Here's how the part is built. I have some questions about the finished solid (model axes, mm). A direction names the side the tool comes from. Coordinates: 2 decimals unless noted, no trailing zeros. Write each loop counter-clockwise with the first axis right and the second up, starting at its lowest first coordinate (ties: lowest second). Pieces come first, ordered by that corner, then holes.
(1) For pin 1 Ø2.5 at (y, z) = (14, 27.51) entering from -X; pin 2 Ø10 at (x, y) = (10.5, 16.5) entering from +Z; pin 3 Ø8 at (x, z) = (12, -0.5) entering from +Y; pin 4 Ø8 at (x, y) = (-25, 17.5) entering from +Z, each with a flat end and sliding along its axis, tell me the tip position at first contact or that it passes through.
(2) Imagine slicing it at D-D, the plane x = 17. List the corners of the cut face in (y, z) for me.
(3) Thinking about a two-plate mould opening in X: for faces 4 (the flat face through (29, 9, 46)), 5 (the flat face through (32.5, 18, 15)), 6 (the flat face through (-16, 4, 17.5)), which applies, released by +X, released by -X, zero draft, split by the parting line, or undercut?
(4) Imagine slicing it at B-B, the plane z = 21. List the corners of the cut face in (x, y) for me.
(5) Please list where these lines run through material, in increasing order: probe 1 along Y at (x, z) = (29.5, 34.5); probe 2 along Y at (x, z) = (-9.5, -12); probe 3 along X at (y, z) = (4.5, 18.5).
(6) Which directions (+Z, -Z, +X, -X, +Y, -Y) give clear straight access to the entire face, cutting with the end or side of a thin tool? Please do faces 1 (the flat face through (-29, 10, 37.5)), 2 (the flat face through (0, 7, -20)), 3 (the flat face through (29, 35, 6.5)).
(7) Imagine slicing it at A-A, the plane y = 19.5. List the corners of the cut face in (x, z) for me, plus the area to 3 significant figures.
(8) Imagine slicing it at C-C, the plane y = 42. List the corners of the cut face in (x, z) for me.
Autodesk Inventor part; units mm, degrees
ref_plane "YZ Plane" through (0, 0, 0) normal (1, 0, 0) x (0, 1, 0)
ref_plane "XZ Plane" through (0, 0, 0) normal (0, 1, 0) x (-1, 0, 0)
ref_plane "XY Plane" through (0, 0, 0) normal (0, 0, 1) x (1, 0, 0)
sketch "Sketch1" plane through (0, 0, 0) normal (0, 1, 0) x (-1, 0, 0)
  line L0 (32.5, 37.5) -> (-32.5, 37.5)
  line L1 (-32.5, 37.5) -> (-32.5, -37.5)
  line L2 (-32.5, -37.5) -> (32.5, -37.5)
  line L3 (32.5, -37.5) -> (32.5, 37.5)
  line L4 (32.5, 37.5) -> (-32.5, -37.5) construction
  line L5 (-32.5, 37.5) -> (32.5, -37.5) construction
  point P0 (0, 0)
  dimension "d0" = 65
  dimension "d1" = 75
extrude "Extrusion1" add sketch "Sketch1" along normal blind 7
sketch "Sketch6" plane through (0, 7, 0) normal (0, 1, 0) x (1, 0, 0)
  line L0 (-32.5, 37.5) -> (-32.5, -37.5)
  line L1 (-32.5, -37.5) -> (-25.5, -37.5)
  line L2 (-32.5, -37.5) -> (32.5, -37.5)
  line L3 (-25.5, -37.5) -> (-25.5, -17.5)
  line L4 (-25.5, -17.5) -> (-5.5, -17.5)
  line L5 (-5.5, -17.5) -> (-5.5, -37.5)
  line L6 (-25.5, -17.5) -> (-32.5, -17.5)
  point P0 (0, 0)
  dimension "d13" = 7
  dimension "d14" = 20
  dimension "d15" = 20
  dimension "d16" = 20
  dimension "d17" = 90
extrude "Extrusion4" cut sketch "Sketch6" against normal blind 14 contours L4 L5 L2 L3
sketch "Sketch7" plane through (0, 7, 0) normal (0, 1, 0) x (1, 0, 0)
  line L0 (-25.5, -37.5) -> (-25.5, -17.5)
  line L1 (-32.5, -37.5) -> (-25.5, -37.5)
  line L2 (-25.5, -37.5) -> (-25.5, -17.5)
  line L3 (-25.5, -17.5) -> (-32.5, -17.5)
  line L4 (-32.5, -17.5) -> (-32.5, -37.5)
  point P0 (0, 0)
extrude "Extrusion5" add sketch "Sketch7" along normal blind 14
sketch "Sketch8" plane through (0, 7, 0) normal (0, 1, 0) x (1, 0, 0)
  line L0 (-5.5, -37.5) -> (32.5, -37.5)
  line L1 (32.5, -37.5) -> (25.5, -37.5)
  line L2 (25.5, -37.5) -> (25.5, 0.5)
  line L3 (25.5, 0.5) -> (32.5, 0.5)
  line L4 (32.5, 0.5) -> (32.5, -37.5)
  point P0 (0, 0)
  dimension "d22" = 7
  dimension "d23" = 38
extrude "Extrusion6" add sketch "Sketch8" along normal blind 18
sketch "Sketch9" plane through (0, 25, 0) normal (0, 1, 0) x (1, 0, 0)
  line L0 (32.5, 0.5) -> (25.5, 0.5)
  line L1 (25.5, 0.5) -> (25.5, -37.5)
  line L2 (32.5, 0.5) -> (25.5, 0.5)
  line L3 (25.5, 0.5) -> (25.5, -6.5)
  line L4 (25.5, -6.5) -> (32.5, -6.5)
  line L5 (32.5, -6.5) -> (32.5, 0.5)
  point P0 (0, 0)
  dimension "d26" = 7
extrude "Extrusion7" add sketch "Sketch9" along normal blind 20
sketch "Sketch10" plane through (0, 25, 0) normal (0, 1, 0) x (1, 0, 0)
  line L0 (32.5, -6.5) -> (32.5, 0.5)
  line L1 (32.5, 0.5) -> (32.5, -54.5)
  line L2 (32.5, -54.5) -> (25.5, -54.5)
  line L3 (25.5, -54.5) -> (25.5, -47.5)
  line L4 (25.5, -47.5) -> (32.5, -47.5)
  line L5 (32.5, -47.5) -> (32.5, -54.5)
  point P0 (0, 0)
  dimension "d29" = 55
  dimension "d30" = 7
  dimension "d31" = 7
extrude "Extrusion8" add sketch "Sketch10" along normal blind 20
sketch "Sketch11" plane through (32.5, 0, 37.5) normal (1, 0, 0) x (0, 0, -1)
  line L0 (-17, 25) -> (-10, 25)
  line L1 (0, 7) -> (0, 25) construction
  line L2 (0, 7) -> (0, 25)
  line L3 (0, 25) -> (-17, 25)
  line L4 (-17, 25) -> (-17, 45)
  line L5 (0, 7) -> (0, 0)
  line L6 (-17, 25) -> (-17, 18)
  line L7 (-17, 18) -> (0, 0)
  point P0 (37.5, 0)
  dimension "d37" = 7
extrude "Extrusion9" add sketch "Sketch11" against normal up to surface (7 mm away)
sketch "Sketch13" plane through (32.5, 0, -37.5) normal (0, 0, -1) x (-1, 0, 0)
  line L0 (65, 7) -> (58, 7)
  line L1 (0, 0) -> (65, 0)
  line L2 (65, 0) -> (65, 7)
  line L3 (65, 7) -> (0, 7)
  line L4 (0, 7) -> (0, 0)
  point P0 (32.5, 0)
extrude "Extrusion10" add sketch "Sketch13" along normal blind 20
sketch "Sketch14" plane through (0, 7, 0) normal (0, 1, 0) x (1, 0, 0)
  point P0 (0, 0)
sketch "Sketch15" plane through (-25.5, 0, 37.5) normal (1, 0, 0) x (0, 0, -1)
  point P0 (37.5, 0)
sketch "Sketch16" plane through (-32.5, 0, 37.5) normal (-1, 0, 0) x (0, 0, 1)
  point P0 (-37.5, 0)
ref_plane "Work Plane1" through (-15.5, 0, 37.5) normal (1, 0, 0) x (0, 0, -1)
mirror "Mirror1" about plane through (-15.5, 0, 37.5) normal (1, 0, 0) of "Extrusion5"
sketch "Sketch18" plane through (-32.5, 0, 37.5) normal (-1, 0, 0) x (0, 0, 1)
  line L0 (-20, 7) -> (-20, 0)
  line L1 (-20, 7) -> (-20, 14)
  line L2 (-20, 7) -> (-20, 21)
  line L3 (-20, 7) -> (-13, 7) construction
  line L4 (-20, 14) -> (-27, 7)
  line L5 (-20, 7) -> (-95, 7)
  point P0 (-37.5, 0)
  dimension "d43" = 7
  dimension "d44" = 90
  dimension "d45" = 45
extrude "Extrusion12" add sketch "Sketch18" against normal up to surface (7 mm away)
mirror "Mirror2" about plane through (-15.5, 0, 37.5) normal (1, 0, 0) of "Extrusion12"
sketch "Sketch19" plane through (-32.5, 0, 37.5) normal (-1, 0, 0) x (0, 0, 1)
  line L0 (0, 0) -> (0, 21)
  line L1 (-20, 14) -> (-20, 21)
  circle A0 centre (-10, 14) radius 1.7 construction
  circle A1 centre (-10, 7) radius 1.7 construction
  point P0 (-37.5, 0)
  dimension "d52" = 3.4
  dimension "d53" = 3.4
sketch "Sketch20" plane through (-32.5, 0, 37.5) normal (-1, 0, 0) x (0, 0, 1)
  line L0 (0, 7) -> (-38, 7)
  circle A0 centre (-9.9905, 7) radius 1.7
  circle A1 centre (-9.9905, 13.9998) radius 1.7
  point P0 (-37.5, 0)
  dimension "d54" = 3.4
  dimension "d55" = 3.4
extrude "Extrusion13" cut sketch "Sketch20" against normal up to surface (34 mm away)
properties part number "graber thingie"
Recorded:
1. pin 1: stops at x = 25.5
1. pin 2: passes through
1. pin 3: stops at y = 7
1. pin 4: stops at z = 37.5
2. outline: (0, -57.5) - (7, -57.5) - (7, 37.5) - (0, 37.5) - close
3. face 4: zero draft
3. face 5: released by +X
3. face 6: undercut
4. outline: (-32.5, 0) - (-25.5, 0) - (-25.5, 21) - (-32.5, 21) - close; (-5.5, 0) - (32.5, 0) - (32.5, 25) - (25.5, 25) - (25.5, 7) - (1.5, 7) - (1.5, 21) - (-5.5, 21) - close
5. probe 1: y = 0 to 25
5. probe 2: y = 0 to 7
5. probe 3: x = -32.5 to -25.5, -5.5 to 32.5
6. face 1: +Z, -X, +Y, -Y
6. face 2: -Z, +Y
6. face 3: +X, -X, +Y
7. outline: (-32.5, 17.5) - (-25.5, 17.5) - (-25.5, 37.5) - (-32.5, 37.5) - close; (-5.5, 17.5) - (1.5, 17.5) - (1.5, 37.5) - (-5.5, 37.5) - close; (25.5, -0.5) - (32.5, -0.5) - (32.5, 54.5) - (25.5, 54.5) - close
7. area: 665 mm2
8. outline: (25.5, -0.5) - (32.5, -0.5) - (32.5, 6.5) - (25.5, 6.5) - close; (25.5, 47.5) - (32.5, 47.5) - (32.5, 54.5) - (25.5, 54.5) - close
